from build123d import *

# Parameters (mm, degrees)
SKETCH1_R           = 15
BOSS_EXTRUDE1_DEPTH = 15
CUT_EXTRUDE1_DEPTH  = 15
SKETCH3_R           = 1.5
CUT_EXTRUDE2_DEPTH  = 15


with BuildPart() as part:
    # Sketch1 → Boss-Extrude1 (new body)
    with BuildSketch(Plane.XY):
        Circle(SKETCH1_R)
    extrude(amount=BOSS_EXTRUDE1_DEPTH)

    # Sketch2 → Cut-Extrude1 (cut)
    with BuildSketch(Plane.XY.offset(15)):
        with BuildLine():
            Line((-1.5, 2), (1.5, 2))
            ThreePointArc((1.5, 2), (0, -2.5), (-1.5, 2))
        make_face()
    extrude(amount=-CUT_EXTRUDE1_DEPTH, mode=Mode.SUBTRACT)

    # Sketch3 → Cut-Extrude2 (cut)
    with BuildSketch(Plane.XY.offset(15)):
        with Locations((0, 9)):
            Circle(SKETCH3_R)
        with Locations((9, 0)):
            Circle(SKETCH3_R)
        with Locations((0, -9)):
            Circle(SKETCH3_R)
        with Locations((-9, 0)):
            Circle(SKETCH3_R)
    extrude(amount=-CUT_EXTRUDE2_DEPTH, mode=Mode.SUBTRACT)


solid = part.part
For this review, take the finished solid that the model builds, in its own axes (mm). Coordinates: 2 decimals unless noted, no trailing zeros. Write each loop counter-clockwise with the first axis right and the second up, starting at its lowest first coordinate (ties: lowest second). Pieces come first, ordered by that corner, then holes. Notation, with made-up numbers: (30, 70) -> (85, 70) arc R22 ccw to (85, 105) -> close; hole circle Ø4 at (28, 24.5). An arc over 180 degrees is marked (long way). Write each question's results on one line, items separated by ' | '. Start each with the question number.
1) Wall thickness on L1, parallel to Y at x = 0, z = 11; L2, parallel to Y at x = -0.75, z = 3.25; L3, parallel to Y at x = -8.5, z = 14: over which ranges is each line inside the solid? List them lowest first. Write a range as [from, to].
2) Consider section A-A (x = 0). Write out the cut boundary in (y, z).
3) The part is to be moulded in two halves that separate along Y. For faces 1 (the face through (-0.325, -10.464, 7.605)), 2 (the face through (3, 0, 15)), 3 (the face through (-14.985, 0.66, 7.395)), 4 (the face through (0, 2, 8)), say which applies: +Y half, -Y half, draft (parallel to the pull), parting line (faces both ways), or undercut.
4) Insertion check: pin 1 (1.5 mm diameter, centred on x = 1, z = 5.5, fed in from -Y); pin 2 (5 mm diameter, centred on x = 9, y = -2.5, fed in from -Z); pin 3 (6 mm diameter, centred on x = 4, z = 10, fed in from +Y); pin 4 (1 mm diameter, centred on x = 2, z = 6.5, fed in from +Y). Each pin has a flat end and moves straight along its axis. Give the tip position at first contact, or say it passes through.
5) Consider section D-D (x = -9). Write out the cut boundary in (y, z), plus the area to 3 significant figures.
6) Consider section B-B (y = 0). Write out the cut boundary in (x, z), plus the area to 3 significant figures.
7) Consider section C-C (z = 3.75). Write out the cut boundary in (x, y), plus the area to 3 significant figures.
Geometry says:
1) L1: [-15, -10.5], [-7.5, -2.5], [2, 7.5], [10.5, 15] | L2: [-14.98, -10.3], [-7.7, -2.38], [2, 7.7], [10.3, 14.98] | L3: [-12.36, -1.41], [1.41, 12.36]
2) outline: (-15, 0) -> (-10.5, 0) -> (-10.5, 15) -> (-15, 15) -> close; (-7.5, 0) -> (-2.5, 0) -> (-2.5, 15) -> (-7.5, 15) -> close; (2, 0) -> (7.5, 0) -> (7.5, 15) -> (2, 15) -> close; (10.5, 0) -> (15, 0) -> (15, 15) -> (10.5, 15) -> close
3) face 1: undercut | face 2: draft | face 3: parting line | face 4: undercut
4) pin 1: y = -15 | pin 2: z = 0 | pin 3: y = 14.97 | pin 4: y = 14.92
5) outline: (-12, 0) -> (-1.5, 0) -> (-1.5, 15) -> (-12, 15) -> close; (1.5, 0) -> (12, 0) -> (12, 15) -> (1.5, 15) -> close | area: 315 mm^2
6) outline: (-15, 0) -> (-10.5, 0) -> (-10.5, 15) -> (-15, 15) -> close; (-7.5, 0) -> (-2.5, 0) -> (-2.5, 15) -> (-7.5, 15) -> close; (2.5, 0) -> (7.5, 0) -> (7.5, 15) -> (2.5, 15) -> close; (10.5, 0) -> (15, 0) -> (15, 15) -> (10.5, 15) -> close | area: 285 mm^2
7) outline: circle Ø30 at (0, 0); hole circle Ø3 at (-9, 0); hole circle Ø3 at (0, -9); hole (-1.5, 2) arc R2.5 ccw (long way) to (1.5, 2) -> close; hole circle Ø3 at (0, 9); hole circle Ø3 at (9, 0) | area: 660 mm^2
